from build123d import *

# Parameters (mm, degrees)
SKETCH1_W           = 115
SKETCH1_H           = 50
BOSS_EXTRUDE1_DEPTH = 205
CUT_EXTRUDE1_DEPTH  = 5


with BuildPart() as part:
    # Sketch1 → Boss-Extrude1 (new body)
    with BuildSketch(Plane.XY):
        with Locations((57.5, 25)):
            Rectangle(SKETCH1_W, SKETCH1_H)
    extrude(amount=BOSS_EXTRUDE1_DEPTH)

    # Sketch2 → Cut-Extrude1 (cut)
    with BuildSketch(Plane.XZ):
        with BuildLine():
            Line((11.75, 179.5), (11.75, 175.5))
            ThreePointArc((11.75, 175.5), (9.75, 173.5), (7.75, 175.5))
            Line((7.75, 175.5), (7.75, 179.5))
            ThreePointArc((7.75, 179.5), (9.75, 181.5), (11.75, 179.5))
        make_face()
        with BuildLine():
            Line((103.25, 179.5), (103.25, 175.5))
            ThreePointArc((103.25, 175.5), (105.25, 173.5), (107.25, 175.5))
            Line((107.25, 175.5), (107.25, 179.5))
            ThreePointArc((107.25, 179.5), (105.25, 181.5), (103.25, 179.5))
        make_face()
        with BuildLine():
            Line((11.75, 7.5), (11.75, 11.5))
            ThreePointArc((11.75, 11.5), (9.75, 13.5), (7.75, 11.5))
            Line((7.75, 11.5), (7.75, 7.5))
            ThreePointArc((7.75, 7.5), (9.75, 5.5), (11.75, 7.5))
        make_face()
        with BuildLine():
            Line((103.25, 7.5), (103.25, 11.5))
            ThreePointArc((103.25, 11.5), (105.25, 13.5), (107.25, 11.5))
            Line((107.25, 11.5), (107.25, 7.5))
            ThreePointArc((107.25, 7.5), (105.25, 5.5), (103.25, 7.5))
        make_face()
    extrude(amount=-CUT_EXTRUDE1_DEPTH, mode=Mode.SUBTRACT)


solid = part.part
Can you work these out from the model? Positions are in its coordinate system, mm. A direction names the side the tool comes from. Round coordinates to 2 decimals unless told otherwise and drop trailing zeros. Use one line per item in the form item = value. Start each with the question number.
Q1. Which directions (+Z, -Z, +X, -X, +Y, -Y) give clear straight access to the entire face, cutting with the end or side of a thin tool? Please do faces 1 (the face through (0, 25, 101)), 2 (the face through (103.25, 2, 178)).
Q2. We'd pull the mould along Z, two halves only. Please class faces 3 (the face through (115, 25, 101)), 4 (the face through (7.75, 2, 10)), 5 (the face through (57, 25, 0)): +Z half, -Z half, draft (parallel to the pull), parting line (faces both ways), or undercut.
Q3. I'm going to push a flat-ended pin straight in: P1, Ø1.2, axis at x = 9, z = 177, coming from the -Y side. Where does the tip first touch, or does it pass through?
Worked out:
q1.face_1 = +Z, -Z, -X, +Y, -Y
q1.face_2 = -Y
q2.face_3 = draft
q2.face_4 = undercut
q2.face_5 = -Z half
q3.P1 = 5
